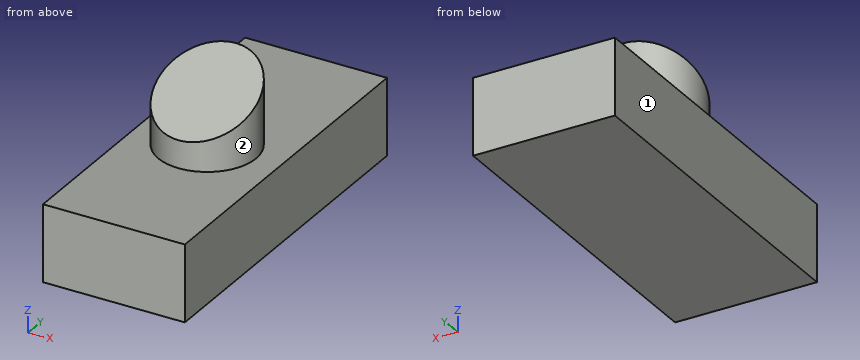
from build123d import *

# Parameters (mm, degrees)
F0_W     = 46.934098
F0_H     = 114.019729
F1_DEPTH = 25.4
F2_R     = 16.172155
F3_DEPTH = 25.4
F5_DEPTH = 46.935098


with BuildPart() as f1:
    # F0 (on Top) → F1 (new body)
    with BuildSketch(Plane.XY):
        with Locations((-23.467049, -4.689149)):
            Rectangle(F0_W, F0_H)
    extrude(amount=F1_DEPTH)

    # F2 (on face) → F3 (join)
    with BuildSketch(Plane.XY.offset(25.4)):
        with Locations((-24.327599, -7.633943)):
            Circle(F2_R)
    extrude(amount=F3_DEPTH)

    # F4 (on face) → F5 (cut, through all)
    with BuildSketch(Plane(origin=(-46.934098, 0, 0), x_dir=(0, -1, 0), z_dir=(-1, 0, 0))):
        Polygon((23.806098, 50.8), (-8.538212, 50.8), (23.806098, 34.50444), align=None)
    extrude(amount=-F5_DEPTH, mode=Mode.SUBTRACT)


solid = f1.part
Build history of the part. All positions in model axes, mm. Face numbers are marked on the shaded views. A direction names the side the tool comes from. Coordinates: 2 decimals unless noted, no trailing zeros. Write each loop counter-clockwise with the first axis right and the second up, starting at its lowest first coordinate (ties: lowest second). Pieces come first, ordered by that corner, then holes.
(1) Cut at A-A on x = -22. List the corners of the cut face in (y, z).
(2) 3-axis set-ups, long thin cutter, end or side, ignore diameter. For the marked faces 1 and 2: which of +Z, -Z, +X, -X, +Y, -Y reach the whole face in a straight line?
(3) Cut at B-B on y = 3. List the corners of the cut face in (x, z).
(4) Pin check, flat tips, straight feed: pin 1 Ø8 at (x, z) = (-15, 33) entering from +Y; pin 2 Ø4 at (x, y) = (-35, 10) entering from +Z; pin 3 Ø23.5 at (x, y) = (-19.5, -14.5) entering from +Z. Stop position of each tip, or through.
(5) Cut at C-C on x = -3.5. List the corners of the cut face in (y, z), and give its area (3 significant figures).
(6) Drill centre lines: line 1 (Z direction, x = -9, y = 11); line 2 (Y direction, x = -13.5, z = 27.5); line 3 (Z direction, x = -26, y = -23.5). Where is each one in solid material? Low to high.
(7) Cut at D-D on z = 39.5. List the corners of the cut face in (x, y), and give its area (3 significant figures).
Working result:
1. outline: (-61.7, 0) - (52.32, 0) - (52.32, 25.4) - (8.37, 25.4) - (8.37, 50.72) - (-23.64, 34.59) - (-23.64, 25.4) - (-61.7, 25.4) - close
2. face 1: +Z, -Z, -X, +Y, -Y
2. face 2: +Z
3. outline: (-46.93, 0) - (0, 0) - (0, 25.4) - (-12.14, 25.4) - (-12.14, 48.01) - (-36.51, 48.01) - (-36.51, 25.4) - (-46.93, 25.4) - close
4. pin 1: stops at y = 7.64
4. pin 2: stops at z = 25.4
4. pin 3: stops at z = 45.11
5. outline: (-61.7, 0) - (52.32, 0) - (52.32, 25.4) - (-61.7, 25.4) - close
5. area: 2,900 mm2
6. line 1: z = 0 to 25.4
6. line 2: y = -19.65 to 4.38
6. line 3: z = 0 to 34.66
7. outline: (-39.24, -13.89) - (-9.41, -13.89) arc R16.17 ccw (long way) to start
7. area: 608 mm2
